from build123d import *

# Parameters (mm, degrees)
SKETCH1_R           = 3.375
BOSS_EXTRUDE1_DEPTH = 20
SKETCH3_W           = 5.1
SKETCH3_H           = 3.1
CUT_EXTRUDE2_DEPTH  = 6
SKETCH2_W           = 4
SKETCH2_H           = 4
BOSS_EXTRUDE2_DEPTH = 5


with BuildPart() as part:
    # Sketch1 → Boss-Extrude1 (new body)
    with BuildSketch(Plane(origin=(0, 0, 0), x_dir=(1, 0, 0), z_dir=(0, 1, 0))):
        with Locations(Location((0, 0, 0), (0, 0, 270))):
            Circle(SKETCH1_R)
    extrude(amount=BOSS_EXTRUDE1_DEPTH)

    # Sketch3 → Cut-Extrude2 (cut)
    with BuildSketch(Plane(origin=(0, 20, 0), x_dir=(1, 0, 0), z_dir=(0, 1, 0))):
        Rectangle(SKETCH3_W, SKETCH3_H)
    extrude(amount=-CUT_EXTRUDE2_DEPTH, mode=Mode.SUBTRACT)

    # Sketch2 → Boss-Extrude2 (add)
    with BuildSketch(Plane(origin=(0, 0, 0), x_dir=(-1, 0, 0), z_dir=(0, -1, 0))):
        Rectangle(SKETCH2_W, SKETCH2_H)
    extrude(amount=BOSS_EXTRUDE2_DEPTH)


solid = part.part
Design review of the part built by this model. Coordinates are the model's own, in mm. A direction names the side the tool comes from. Give positions to 0.01 mm unless a question says otherwise; leave off trailing zeros. Loops run counter-clockwise (first coordinate to the right, second up) from the corner with the lowest first, then second, coordinate; pieces in that order, holes last. Notation, with made-up numbers: (31, 89) - (43, 89) arc R33 ccw to (43, 117) - close; hole circle Ø8 at (-12.5, -30.5). An arc over 180 degrees is marked (long way). Write item = value, one per line.
1) Tool access review of faces 1 (the face through (2, -2, 0)), 2 (the face through (0, -2, 2)), 3 (the face through (0, -2, -2)), 4 (the face through (0, 17, -1.55)): name each direction out of +Z, -Z, +X, -X, +Y, -Y from which nothing blocks a thin tool from reaching the whole face with its end or side.
Result sheet:
face_1 = +Z, -Z, +X, -Y
face_2 = +Z, +X, -X, -Y
face_3 = -Z, +X, -X, -Y
face_4 = +Y
2) Take a section at B-B on x = 0. State the section outline as (y, z) points (3 decimals).
Result sheet:
outline = (-5, -2) - (0, -2) - (0, -3.375) - (20, -3.375) - (20, -1.55) - (14, -1.55) - (14, 1.55) - (20, 1.55) - (20, 3.375) - (0, 3.375) - (0, 2) - (-5, 2) - close
3) Take a section at D-D on y = 6.75. State the section outline as (x, z) points (3 decimals), and give its area (3 significant figures).
Result sheet:
outline = circle Ø6.75 at (0, 0)
area = 35.8 mm2
4) Clearance check with flat-ended pins moving along their axes: pin 1 Ø1.5 at (x, y) = (-1, 13.5) entering from +Z; pin 2 Ø1.5 at (x, z) = (-1.5, -0.5) entering from +Y; pin 3 Ø1.2 at (x, y) = (0, -2) entering from +Z. State where each tip first meets the part, or that it passes through.
Result sheet:
pin_1 = 3.37
pin_2 = 14
pin_3 = 2
5) To check wall thickness, follow line 1 (X direction, y = 18.5, z = 0) (3 decimals); line 2 (Y direction, x = 2.75, z = -1.75); line 3 (X direction, y = -3.25, z = 1.75). State the ranges of each line that lie inside material, in increasing order.
Result sheet:
line_1 = -3.375 to -2.55, 2.55 to 3.375
line_2 = 0 to 20
line_3 = -2 to 2
6) Take a section at C-C on y = 14.75. State the section outline as (x, z) points (3 decimals), and give its area (3 significant figures).
Result sheet:
outline = circle Ø6.75 at (0, 0); hole (-2.55, -1.55) - (2.55, -1.55) - (2.55, 1.55) - (-2.55, 1.55) - close
area = 20.0 mm2
7) Draft analysis for pull direction Z (two halves, no side actions). For faces 5 (the face through (-2, -2, 0)), 6 (the face through (0, 14, 0)), 7 (the face through (2.55, 17, 0)), 8 (the face through (-3.3, 9.9, -0.7)), state which applies: +Z half, -Z half, draft (parallel to the pull), parting line (faces both ways), or undercut.
Result sheet:
face_5 = draft
face_6 = undercut
face_7 = undercut
face_8 = parting line
8) Take a section at A-A on z = 0. State the section outline as (x, y) points (3 decimals), and give its area (3 significant figures).
Result sheet:
outline = (-3.375, 0) - (-2, 0) - (-2, -5) - (2, -5) - (2, 0) - (3.375, 0) - (3.375, 20) - (2.55, 20) - (2.55, 14) - (-2.55, 14) - (-2.55, 20) - (-3.375, 20) - close
area = 124 mm2
